Here's how the part is built. I have some questions about the finished solid (model axes, mm). Face numbers are marked on the shaded views. Round coordinates to 2 decimals unless told otherwise and drop trailing zeros. Loops run counter-clockwise (first coordinate to the right, second up) from the corner with the lowest first, then second, coordinate; pieces in that order, holes last. Notation, with made-up numbers: M 26.5,-17 L 60.5,-17 A22 cw 60.5,-2 Z; hole C 61.25,60 d7. An arc over 180 degrees is marked long. Use a Markdown table: item, result.
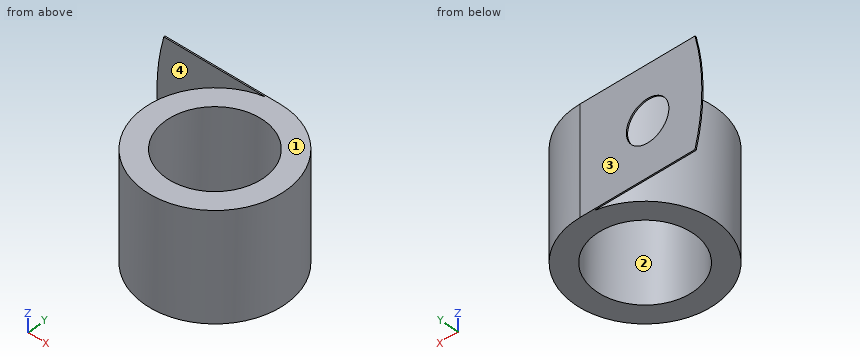
```python
from build123d import *

# Parameters (mm, degrees)
SKETCH1_R           = 8.255
SKETCH1_R_2         = 5.715
BOSS_EXTRUDE1_DEPTH = 6.35
CUT_EXTRUDE1_REACH  = 18.51
SKETCH5_R           = 2.4892


with BuildPart() as part:
    # Sketch1 → Boss-Extrude1 (new body, symmetric)
    with BuildSketch(Plane.XY):
        Circle(SKETCH1_R)
        Circle(SKETCH1_R_2, mode=Mode.SUBTRACT)
        with BuildLine():
            ThreePointArc((-1.578891459, 8.1026), (-0.793114746, 8.216811669), (0, 8.255))
            Line((0, 8.255), (-14.278891459, 8.255))
            Line((-14.278891459, 8.255), (-14.278891459, 8.1026))
            Line((-14.278891459, 8.1026), (-1.578891459, 8.1026))
        make_face()
    extrude(amount=BOSS_EXTRUDE1_DEPTH, both=True)

    # Sketch5 → Cut-Extrude1 (cut, up to next)
    with BuildSketch(Plane(origin=(0, 8.255, 0), x_dir=(1, 0, 0), z_dir=(0, 1, 0)), mode=Mode.PRIVATE) as cut_extrude1_sk1:
        with BuildLine():
            ThreePointArc((-14.278891459, -1.01e-07), (-14.076445751, 3.200508979), (-13.472335708, 6.35))
            Line((-13.472335708, 6.35), (-14.278891459, 6.35))
            Line((-14.278891459, 6.35), (-14.278891459, -1.01e-07))
        make_face()
    cut_extrude1_tool1 = extrude(cut_extrude1_sk1.sketch, amount=-CUT_EXTRUDE1_REACH, mode=Mode.PRIVATE) & part.part
    add(cut_extrude1_tool1.solids().sort_by_distance((-14.037598, 8.255, -4.767585))[0], mode=Mode.SUBTRACT)
    # Sketch5 → Cut-Extrude1 (cut, up to next)
    with BuildSketch(Plane(origin=(0, 8.255, 0), x_dir=(1, 0, 0), z_dir=(0, 1, 0)), mode=Mode.PRIVATE) as cut_extrude1_sk2:
        with BuildLine():
            ThreePointArc((-13.472335708, -6.35), (-14.076445738, -3.200509079), (-14.278891459, -1.01e-07))
            Line((-14.278891459, -1.01e-07), (-14.278891459, -6.35))
            Line((-14.278891459, -6.35), (-13.472335708, -6.35))
        make_face()
    cut_extrude1_tool2 = extrude(cut_extrude1_sk2.sketch, amount=-CUT_EXTRUDE1_REACH, mode=Mode.PRIVATE) & part.part
    add(cut_extrude1_tool2.solids().sort_by_distance((-14.037598, 8.255, 4.767585))[0], mode=Mode.SUBTRACT)
    # Sketch5 → Cut-Extrude1 (cut, up to next)
    with BuildSketch(Plane(origin=(0, 8.255, 0), x_dir=(1, 0, 0), z_dir=(0, 1, 0)), mode=Mode.PRIVATE) as cut_extrude1_sk3:
        with Locations((-7.928891459, 0)):
            Circle(SKETCH5_R)
    cut_extrude1_tool3 = extrude(cut_extrude1_sk3.sketch, amount=-CUT_EXTRUDE1_REACH, mode=Mode.PRIVATE) & part.part
    add(cut_extrude1_tool3.solids().sort_by_distance((-7.928891, 8.255, 0))[0], mode=Mode.SUBTRACT)


solid = part.part
```
Q1. Imagine slicing it at B-B, the plane z = -1. Please give me the cut outline in (x, y) (3 decimals), then the cut area to 3 significant figures.
Return value:
| item | result |
|---|---|
| outline | M -14.259,8.103 L -10.208,8.103 L -10.208,8.255 L -14.259,8.255 Z; M -5.649,8.103 L -1.579,8.103 A8.255 ccw long 0,8.255 L -5.649,8.255 Z; hole C 0,0 d11.43 |
| area | 113 mm^2 |
Q2. Imagine slicing it at D-D, the plane z = -2.75. Please give me the cut outline in (x, y) (3 decimals), then the cut area to 3 significant figures.
Return value:
| item | result |
|---|---|
| outline | M -14.13,8.103 L -1.579,8.103 A8.255 ccw long 0,8.255 L -14.13,8.255 Z; hole C 0,0 d11.43 |
| area | 113 mm^2 |
Q3. Imagine slicing it at C-C, the plane x = -8. Please give me the cut outline in (y, z) (3 decimals).
Return value:
| item | result |
|---|---|
| outline | M -2.036,-6.35 L 2.036,-6.35 L 2.036,6.35 L -2.036,6.35 Z; M 8.103,-6.35 L 8.255,-6.35 L 8.255,-2.488 L 8.103,-2.488 Z; M 8.103,2.488 L 8.255,2.488 L 8.255,6.35 L 8.103,6.35 Z |
Q4. Will these pins go through, and if not, where does the flat tip stop? P1, Ø1.5, axis at y = -2.5, z = 2, coming from the +X side; P2, Ø5, axis at y = -4.5, z = 5, coming from the -X side; P3, Ø5.5, axis at x = -7.93, z = 0, coming from the -Y side.
Return value:
| item | result |
|---|---|
| P1 | stops at x = 8.07 |
| P2 | stops at x = -8.01 |
| P3 | stops at y = -6.43 |
Q5. Imagine slicing it at A-A, the plane y = 0. Please give me the cut outline in (x, z) (3 decimals), then the cut area to 3 significant figures.
Return value:
| item | result |
|---|---|
| outline | M -8.255,-6.35 L -5.715,-6.35 L -5.715,6.35 L -8.255,6.35 Z; M 5.715,-6.35 L 8.255,-6.35 L 8.255,6.35 L 5.715,6.35 Z |
| area | 64.5 mm^2 |
Q6. We'd pull the mould along Y, two halves only. Please class the marked faces 1, 2, 3 and 4: pulls with the +Y half, pulls with the -Y half, needs draft (parallel to the pull), parting line crosses it, or undercut.
Return value:
| item | result |
|---|---|
| face 1 | needs draft |
| face 2 | undercut |
| face 3 | pulls with the +Y half |
| face 4 | undercut |
Q7. I need wall thicknesses on line 1 (Y direction, x = -7, z = -5) (1 decimal); line 2 (Y direction, x = 2.5, z = 5); line 3 (X direction, y = 4.75, z = 4). Which ranges of each line are inside material? Lowest first, please. Write a range as from..to.
Return value:
| item | result |
|---|---|
| line 1 | y = -4.4..4.4, 8.1..8.3 |
| line 2 | y = -7.87..-5.14, 5.14..7.87 |
| line 3 | x = -6.75..-3.18, 3.18..6.75 |
